from build123d import *

# Parameters (mm, degrees)
F1_DEPTH = 25.4
F2_R     = 1.651
F3_DEPTH = 25.4


with BuildPart() as f1:
    # F0 (on Top) → F1 (new body)
    with BuildSketch(Plane.XY):
        with BuildLine():
            ThreePointArc((12.886483, -3.666521), (13.269461, -1.851011), (13.397941, 0))
            ThreePointArc((13.397941, 0), (13.39761, 0.094267), (13.396615, 0.18853))
            ThreePointArc((13.396615, 0.18853), (13.37896, 0.712915), (13.340788, 1.236206))
            ThreePointArc((13.340788, 1.236206), (13.02016, 3.159153), (12.423866, 5.015214))
            ThreePointArc((12.423866, 5.015214), (12.217975, 5.497811), (11.993345, 5.971976))
            ThreePointArc((11.993345, 5.971976), (10.99972, 7.649247), (9.773206, 9.164566))
            ThreePointArc((9.773206, 9.164566), (9.406884, 9.540198), (9.026135, 9.901198))
            ThreePointArc((9.026135, 9.901198), (7.493707, 11.106268), (5.80262, 12.076193))
            ThreePointArc((5.80262, 12.076193), (5.325341, 12.294128), (4.839895, 12.493208))
            ThreePointArc((4.839895, 12.493208), (2.975627, 13.063326), (1.048358, 13.356862))
            ThreePointArc((1.048358, 13.356862), (0.524581, 13.387668), (0, 13.397941))
            ThreePointArc((0, 13.397941), (-1.944328, 13.256109), (-3.84749, 12.833614))
            ThreePointArc((-3.84749, 12.833614), (-4.347026, 12.673129), (-4.839895, 12.493208))
            ThreePointArc((-4.839895, 12.493208), (-6.601691, 11.658581), (-8.223714, 10.577115))
            ThreePointArc((-8.223714, 10.577115), (-8.631543, 10.247014), (-9.026135, 9.901198))
            ThreePointArc((-9.026135, 9.901198), (-10.367458, 8.486497), (-11.489279, 6.892118))
            ThreePointArc((-11.489279, 6.892118), (-11.750323, 6.436983), (-11.993345, 5.971976))
            ThreePointArc((-11.993345, 5.971976), (-12.733043, 4.168265), (-13.203154, 2.276302))
            ThreePointArc((-13.203154, 2.276302), (-13.282156, 1.757602), (-13.340788, 1.236206))
            ThreePointArc((-13.340788, 1.236206), (-13.37896, -0.712915), (-13.13387, -2.646941))
            ThreePointArc((-13.13387, -2.646941), (-13.02016, -3.159153), (-12.886483, -3.666521))
            ThreePointArc((-12.886483, -3.666521), (-12.217975, -5.497811), (-11.290783, -7.2127))
            ThreePointArc((-11.290783, -7.2127), (-10.99972, -7.649247), (-10.691788, -8.074063))
            ThreePointArc((-10.691788, -8.074063), (-9.406884, -9.540198), (-7.922814, -10.804344))
            ThreePointArc((-7.922814, -10.804344), (-7.493707, -11.106268), (-7.053107, -11.391159))
            ThreePointArc((-7.053107, -11.391159), (-5.325341, -12.294128), (-3.484825, -12.936801))
            ThreePointArc((-3.484825, -12.936801), (-2.975627, -13.063326), (-2.461865, -13.169816))
            ThreePointArc((-2.461865, -13.169816), (-0.524581, -13.387668), (1.423809, -13.322072))
            ThreePointArc((1.423809, -13.322072), (1.944328, -13.256109), (2.461865, -13.169816))
            ThreePointArc((2.461865, -13.169816), (4.347026, -12.673129), (6.14015, -11.908123))
            ThreePointArc((6.14015, -11.908123), (6.601691, -11.658581), (7.053107, -11.391159))
            ThreePointArc((7.053107, -11.391159), (8.631543, -10.247014), (10.027229, -8.885916))
            ThreePointArc((10.027229, -8.885916), (10.367458, -8.486497), (10.691788, -8.074063))
            ThreePointArc((10.691788, -8.074063), (11.750323, -6.436983), (12.560076, -4.663617))
            ThreePointArc((12.560076, -4.663617), (12.733043, -4.168265), (12.886483, -3.666521))
        make_face()
        with BuildLine():
            Line((15.135725, -17.13642), (10.027229, -8.885916))
            ThreePointArc((10.027229, -8.885916), (8.631543, -10.247014), (7.053107, -11.391159))
            Line((7.053107, -11.391159), (11.864523, -19.161862))
            ThreePointArc((11.864523, -19.161862), (14.512845, -19.784742), (15.135725, -17.13642))
        make_face()
        with BuildLine():
            Line((20.304032, -10.511581), (12.560076, -4.663617))
            ThreePointArc((12.560076, -4.663617), (11.750323, -6.436983), (10.691788, -8.074063))
            Line((10.691788, -8.074063), (17.985401, -13.581944))
            ThreePointArc((17.985401, -13.581944), (20.679898, -13.206078), (20.304032, -10.511581))
        make_face()
        with BuildLine():
            ThreePointArc((13.396615, 0.18853), (13.39761, 0.094267), (13.397941, 0))
            ThreePointArc((13.397941, 0), (13.269461, -1.851011), (12.886483, -3.666521))
            Line((12.886483, -3.666521), (21.677251, -6.16771))
            ThreePointArc((21.677251, -6.16771), (24.054016, -4.84386), (22.730167, -2.467095))
            Line((22.730167, -2.467095), (13.396615, 0.18853))
        make_face()
        with BuildLine():
            ThreePointArc((12.423866, 5.015214), (13.02016, 3.159153), (13.340788, 1.236206))
            Line((13.340788, 1.236206), (22.441468, 2.079508))
            ThreePointArc((22.441468, 2.079508), (24.179506, 4.172548), (22.086467, 5.910586))
            Line((22.086467, 5.910586), (12.423866, 5.015214))
        make_face()
        with BuildLine():
            ThreePointArc((9.773206, 9.164566), (10.99972, 7.649247), (11.993345, 5.971976))
            Line((11.993345, 5.971976), (20.174841, 10.045877))
            ThreePointArc((20.174841, 10.045877), (21.03942, 12.62543), (18.459867, 13.490009))
            Line((18.459867, 13.490009), (9.773206, 9.164566))
        make_face()
        with BuildLine():
            ThreePointArc((5.80262, 12.076193), (7.493707, 11.106268), (9.026135, 9.901198))
            Line((9.026135, 9.901198), (15.18349, 16.655495))
            ThreePointArc((15.18349, 16.655495), (15.057844, 19.373178), (12.34016, 19.247532))
            Line((12.34016, 19.247532), (5.80262, 12.076193))
        make_face()
        with BuildLine():
            ThreePointArc((1.048358, 13.356862), (2.975627, 13.063326), (4.839895, 12.493208))
            Line((4.839895, 12.493208), (8.141524, 21.015695))
            ThreePointArc((8.141524, 21.015695), (7.042622, 23.504471), (4.553846, 22.405569))
            Line((4.553846, 22.405569), (1.048358, 13.356862))
        make_face()
        with BuildLine():
            ThreePointArc((-3.84749, 12.833614), (-1.944328, 13.256109), (0, 13.397941))
            Line((0, 13.397941), (0, 22.53761))
            ThreePointArc((0, 22.53761), (-1.923745, 24.461355), (-3.84749, 22.53761))
            Line((-3.84749, 22.53761), (-3.84749, 12.833614))
        make_face()
        with BuildLine():
            ThreePointArc((-8.223714, 10.577115), (-6.601691, 11.658581), (-4.839895, 12.493208))
            Line((-4.839895, 12.493208), (-8.141524, 21.015695))
            ThreePointArc((-8.141524, 21.015695), (-10.6303, 22.114597), (-11.729202, 19.625822))
            Line((-11.729202, 19.625822), (-8.223714, 10.577115))
        make_face()
        with BuildLine():
            ThreePointArc((-11.489279, 6.892118), (-10.367458, 8.486497), (-9.026135, 9.901198))
            Line((-9.026135, 9.901198), (-15.18349, 16.655495))
            ThreePointArc((-15.18349, 16.655495), (-17.901173, 16.781141), (-18.026819, 14.063457))
            Line((-18.026819, 14.063457), (-11.489279, 6.892118))
        make_face()
        with BuildLine():
            ThreePointArc((-13.203154, 2.276302), (-12.733043, 4.168265), (-11.993345, 5.971976))
            Line((-11.993345, 5.971976), (-20.174841, 10.045877))
            ThreePointArc((-20.174841, 10.045877), (-22.754394, 9.181298), (-21.889815, 6.601745))
            Line((-21.889815, 6.601745), (-13.203154, 2.276302))
        make_face()
        with BuildLine():
            Line((-22.79647, -1.751569), (-13.13387, -2.646941))
            ThreePointArc((-13.13387, -2.646941), (-13.37896, -0.712915), (-13.340788, 1.236206))
            Line((-13.340788, 1.236206), (-22.441468, 2.079508))
            ThreePointArc((-22.441468, 2.079508), (-24.534508, 0.34147), (-22.79647, -1.751569))
        make_face()
        with BuildLine():
            Line((-20.624335, -9.868325), (-11.290783, -7.2127))
            ThreePointArc((-11.290783, -7.2127), (-12.217975, -5.497811), (-12.886483, -3.666521))
            Line((-12.886483, -3.666521), (-21.677251, -6.16771))
            ThreePointArc((-21.677251, -6.16771), (-23.001101, -8.544475), (-20.624335, -9.868325))
        make_face()
        with BuildLine():
            Line((-15.66677, -16.652308), (-7.922814, -10.804344))
            ThreePointArc((-7.922814, -10.804344), (-9.406884, -9.540198), (-10.691788, -8.074063))
            Line((-10.691788, -8.074063), (-17.985401, -13.581944))
            ThreePointArc((-17.985401, -13.581944), (-18.361267, -16.276442), (-15.66677, -16.652308))
        make_face()
        with BuildLine():
            Line((-8.593321, -21.187305), (-3.484825, -12.936801))
            ThreePointArc((-3.484825, -12.936801), (-5.325341, -12.294128), (-7.053107, -11.391159))
            Line((-7.053107, -11.391159), (-11.864523, -19.161862))
            ThreePointArc((-11.864523, -19.161862), (-11.241643, -21.810185), (-8.593321, -21.187305))
        make_face()
        with BuildLine():
            Line((-0.359295, -22.860839), (1.423809, -13.322072))
            ThreePointArc((1.423809, -13.322072), (-0.524581, -13.387668), (-2.461865, -13.169816))
            Line((-2.461865, -13.169816), (-4.141275, -22.153864))
            ThreePointArc((-4.141275, -22.153864), (-2.603772, -24.398341), (-0.359295, -22.860839))
        make_face()
        with BuildLine():
            Line((7.923254, -21.44689), (6.14015, -11.908123))
            ThreePointArc((6.14015, -11.908123), (4.347026, -12.673129), (2.461865, -13.169816))
            Line((2.461865, -13.169816), (4.141275, -22.153864))
            ThreePointArc((4.141275, -22.153864), (6.385752, -23.691367), (7.923254, -21.44689))
        make_face()
    extrude(amount=F1_DEPTH)

    # F2 (on face) → F3 (cut)
    with BuildSketch(Plane.XY.offset(25.4)):
        Circle(F2_R)
    extrude(amount=-F3_DEPTH, mode=Mode.SUBTRACT)


solid = f1.part
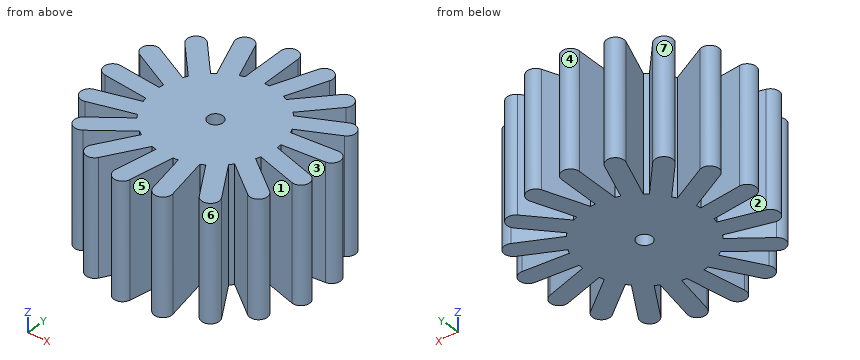
Model file for the job. Use its own axes, mm. Face numbers are marked on the shaded views. A direction names the side the tool comes from. Give positions to 0.01 mm unless a question says otherwise; leave off trailing zeros. Order: outer loops, then holes, each group sorted by start corner. A loop starts at its lowest first (then second) coordinate and runs counter-clockwise, first axis right, second up. Notation, with made-up numbers: (45.25, -4.5) - (72.25, -4.5) arc R5 cw to (72.25, 3.5) - close; hole circle Ø9 at (77, 4.25). An arc over 180 degrees is marked (long way). Return JSON: item names as keys, results as strings.
1) Flat gauge pins, fed straight in: P1, Ø8, axis at x = -11.5, z = 9, coming from the +Y side; P2, Ø8, axis at x = 17, z = 15, coming from the +Y side; P3, Ø10, axis at x = 13.5, y = 9.5, coming from the -Z side; P4, Ø7.5, axis at y = 18, z = 18, coming from the +X side. Where does each tip first touch, or does it go through?
Geometry says:
{"P1": "y = 22.24", "P2": "y = 19.88", "P3": "z = 0", "P4": "x = 15.69"}
2) Pull direction Y, two halves, no side cores. Call the marked faces 4, 5, 6 and 7: pulls with the +Y half, pulls with the -Y half, needs draft (parallel to the pull), parting line crosses it, or undercut.
Geometry says:
{"face 4": "pulls with the +Y half", "face 5": "pulls with the -Y half", "face 6": "undercut", "face 7": "undercut"}
3) 3-axis set-ups, long thin cutter, end or side, ignore diameter. For the marked faces 1, 2 and 3: which of +Z, -Z, +X, -X, +Y, -Y reach the whole face in a straight line?
Geometry says:
{"face 1": "+Z, -Z", "face 2": "+Z, -Z, -X", "face 3": "+Z, -Z, +X"}
4) Cut at C-C, the plane x = -14. Give the cut face in (y, z), plus the area to 3 significant figures.
Geometry says:
{"outline": "(-15.39, 0) - (-10.57, 0) - (-10.57, 25.4) - (-15.39, 25.4) - close; (-7.98, 0) - (-3.98, 0) - (-3.98, 25.4) - (-7.98, 25.4) - close; (-2.57, 0) - (1.3, 0) - (1.3, 25.4) - (-2.57, 25.4) - close; (2.67, 0) - (6.97, 0) - (6.97, 25.4) - (2.67, 25.4) - close; (9.65, 0) - (15.36, 0) - (15.36, 25.4) - (9.65, 25.4) - close", "area": "576 mm²"}
5) Probe line 1 (X direction, y = -19.5, z = 24.75); line 2 (Y direction, x = 20.5, z = 13.75); line 3 (X direction, y = 1, z = 9.25). List the from-to ranges inside material, lowest first. Write a range as from..to.
Geometry says:
{"line 1": "-12.03..-7.55, -3.65..0.27, 3.65..7.56, 12.13..14.87", "line 2": "-13.41..-10.68, -5.83..-1.83, 1.9..5.76, 10.25..13.29", "line 3": "-24.35..-1.31, 1.31..13.36"}
6) Cut at A-A, the plane x = 16.5. Give the cut face in (y, z), plus the area to 3 significant figures.
Geometry says:
{"outline": "(-12.46, 0) - (-7.64, 0) - (-7.64, 25.4) - (-12.46, 25.4) - close; (-4.69, 0) - (-0.69, 0) - (-0.69, 25.4) - (-4.69, 25.4) - close; (1.53, 0) - (5.39, 0) - (5.39, 25.4) - (1.53, 25.4) - close; (8.22, 0) - (12.51, 0) - (12.51, 25.4) - (8.22, 25.4) - close", "area": "431 mm²"}
7) Cut at B-B, the plane y = 18.5. Give the cut face in (x, z), plus the area to 3 significant figures.
Geometry says:
{"outline": "(-11.29, 0) - (-7.17, 0) - (-7.17, 25.4) - (-11.29, 25.4) - close; (-3.85, 0) - (0, 0) - (0, 25.4) - (-3.85, 25.4) - close; (3.04, 0) - (7.17, 0) - (7.17, 25.4) - (3.04, 25.4) - close; (11.66, 0) - (15.61, 0) - (15.61, 25.4) - (11.66, 25.4) - close", "area": "408 mm²"}
